```python
from build123d import *

# Parameters (mm, degrees)
F0_W     = 62
F0_H     = 8
F0_W_2   = 56
F0_H_2   = 2
F1_DEPTH = 86
F2_W     = 62
F2_H     = 15
F3_DEPTH = 5
F4_W     = 62
F4_H     = 2
F5_DEPTH = 4
F6_R     = 3


with BuildPart() as f1:
    # F0 (on Top) → F1 (new body)
    with BuildSketch(Plane.XY):
        Rectangle(F0_W, F0_H)
        Rectangle(F0_W_2, F0_H_2, mode=Mode.SUBTRACT)
    extrude(amount=F1_DEPTH)

    # F2 (on Front) → F3 (cut)
    with BuildSketch(Plane.XZ):
        with Locations((0, 78.5)):
            Rectangle(F2_W, F2_H)
    extrude(amount=-F3_DEPTH, mode=Mode.SUBTRACT)

    # F4 (on Front) → F5 (join, symmetric)
    with BuildSketch(Plane.XZ):
        with Locations((0, -1)):
            Rectangle(F4_W, F4_H)
    extrude(amount=F5_DEPTH, both=True)

    # F6
    f6_edges = [f1.edges().sort_by_distance(p)[0] for p in [
        (0, 4, -2),
        (0, -4, -2),
        (31, 0, -2),
        (-31, 0, -2),
        (31, 4, 34.5),
        (31, -4, 42),
        (-31, 4, 34.5),
        (-31, -4, 42),
    ]]
    fillet(f6_edges, radius=F6_R)


solid = f1.part
```
The listing builds one solid part. Answer for the finished solid, in the listing's coordinates (mm). A direction names the side the tool comes from. Coordinates: 2 decimals unless noted, no trailing zeros. Loops run counter-clockwise (first coordinate to the right, second up) from the corner with the lowest first, then second, coordinate; pieces in that order, holes last. Notation, with made-up numbers: M 69,-9 L 94,-9 A22 cw 94,15 Z; hole C 65,59 d1. An arc over 180 degrees is marked long. Answer as CSV lines item,"result". Start each with the question number.
(1) The mould has two halves that part along Y. Classify faces 1 (the flat face through (0, 0, 0)), 2 (the flat face through (0, -1, 42)), 3 (the flat face through (29, 0, 79)), 4 (the cylindrical face through (-30.14, -0.01, -1.1)): pulls with the +Y half, pulls with the -Y half, needs draft (parallel to the pull), parting line crosses it, or undercut.
(2) For faces 5 (the flat face through (-30, 0, 79)), 6 (the flat face through (0, 1, 35)), 7 (the cylindrical face through (0.39, 3.14, -1.1)), determine the directions among +Z, -Z, +X, -X, +Y, -Y from which every point of the face is accessible in a straight line to the end or side of a thin tool.
(3) The part is cut by section C-C (y = -2.5). Give the vertices of the cut face in (x, z), and give its area (3 significant figures).
(4) Given pin 1 (0.6 mm diameter, centred on x = 2, y = -0.5, fed in from +Z); pin 2 (1.5 mm diameter, centred on y = 2, z = 32.5, fed in from -X); pin 3 (0.9 mm diameter, centred on x = -29, z = 77, fed in from +Y); pin 4 (2 mm diameter, centred on y = -1.5, z = 62, fed in from +X), each flat-ended and moving along its own axis, determine where each tip first touches the part or whether it passes through.
(5) The part is cut by section A-A (z = 49). Give the vertices of the cut face in (x, y).
(6) Find the intervals of material crossed by L1, parallel to X at y = 0, z = 16.5; L2, parallel to Y at x = 23.5, z = 3.5; L3, parallel to Z at x = 10.5, y = 0, in increasing order. Write a range as [from, to].
(7) The part is cut by section B-B (x = -8.5). Give the vertices of the cut face in (y, z), and give its area (3 significant figures).
Determined:
1,face 1,"undercut"
1,face 2,"undercut"
1,face 3,"pulls with the +Y half"
1,face 4,"needs draft"
2,face 5,"+Z, +X, -X, +Y"
2,face 6,"+Z"
2,face 7,"-Z, +X, -X, +Y"
3,outline,"M -30.6,1 A2.6 ccw -28,-1.6 L 28,-1.6 A2.6 ccw 30.6,1 L 30.6,86 L -30.6,86 Z"
3,area,"5,360 mm2"
4,pin 1,"z = 0"
4,pin 2,"x = -30.99"
4,pin 3,"y = 0"
4,pin 4,"x = 31"
5,outline,"M -31,-1 A3 ccw -28,-4 L 28,-4 A3 ccw 31,-1 L 31,1 A3 ccw 28,4 L -28,4 A3 ccw -31,1 Z; hole M -28,-1 L 28,-1 L 28,1 L -28,1 Z"
6,L1,"[-31, -28], [28, 31]"
6,L2,"[-4, -1], [1, 4]"
6,L3,"[-2, 0]"
7,outline,"M -4,1 A3 ccw -1,-2 L 1,-2 A3 ccw 4,1 L 4,71 L 1,71 L 1,0 L -1,0 L -1,86 L -4,86 Z"
7,area,"483 mm2"
